Could you check a few things on this model? Use its own coordinates, in mm. A direction names the side the tool comes from. Give positions to 0.01 mm unless a question says otherwise; leave off trailing zeros. Loops run counter-clockwise (first coordinate to the right, second up) from the corner with the lowest first, then second, coordinate; pieces in that order, holes last. Notation, with made-up numbers: M 18,61.25 L 69,61.25 A9 cw 69,75.25 Z; hole C 2,-18 d7. An arc over 180 degrees is marked long. Write each question's results on one line, items separated by ' | '. Start each with the question number.
from build123d import *

# Parameters (mm, degrees)
SKETCH042_W     = 20
SKETCH042_H     = 20
PAD022_DEPTH    = 9
SKETCH043_R     = 7
PAD023_DEPTH    = 10
POCKET023_DEPTH = 8
SKETCH046_W     = 8.75
SKETCH046_H     = 5.2
POCKET024_DEPTH = 1
SKETCH047_R     = 3.7
POCKET025_DEPTH = 3
SKETCH048_R     = 1.675
POCKET026_DEPTH = 5
FILLET007_R     = 2
POCKET033_DEPTH = 5.2
SKETCH058_R     = 1.7
POCKET034_DEPTH = 10


with BuildPart() as part:
    # Sketch042 → Pad022 (new body)
    with BuildSketch(Plane.XZ):
        with Locations((-19.773271, -18.660706)):
            Rectangle(SKETCH042_W, SKETCH042_H)
    extrude(amount=PAD022_DEPTH)

    # Sketch043 (on Face6 of Pad022) → Pad023 (join)
    with BuildSketch(Plane.XZ.offset(9)):
        with Locations((-19.773271, -18.660706)):
            Circle(SKETCH043_R)
    extrude(amount=PAD023_DEPTH)

    # Sketch044 (on Face8 of Pad023) → Pocket023 (cut)
    with BuildSketch(Plane.XZ.offset(19)):
        with BuildLine():
            Line((-17.123271, -18.660706), (-17.123271, -31.745383))
            Line((-17.123271, -31.745383), (-22.423271, -31.745383))
            Line((-22.423271, -31.745383), (-22.423271, -18.660706))
            ThreePointArc((-17.123271, -18.660706), (-19.773271, -16.010706), (-22.423271, -18.660706))
        make_face()
    extrude(amount=-POCKET023_DEPTH, mode=Mode.SUBTRACT)

    # Sketch046 (on Face6 of Pocket023) → Pocket024 (cut)
    with BuildSketch(Plane(origin=(0, 0, -28.660706), x_dir=(1, 0, 0), z_dir=(0, 0, -1))):
        with Locations((-19.773271, 11.6)):
            Rectangle(SKETCH046_W, SKETCH046_H)
    extrude(amount=-POCKET024_DEPTH, mode=Mode.SUBTRACT)

    # Sketch047 (on Face4 of Pocket024) → Pocket025 (cut)
    with BuildSketch(Plane(origin=(0, 0, 0), x_dir=(1, 0, 0), z_dir=(0, 1, 0))):
        with Locations((-19.773271, 18.660706)):
            Circle(SKETCH047_R)
    extrude(amount=-POCKET025_DEPTH, mode=Mode.SUBTRACT)

    # Sketch048 (on Face11 of Pocket025) → Pocket026 (cut)
    with BuildSketch(Plane.XZ.offset(19)):
        with Locations((-19.773271, -18.660706)):
            Circle(SKETCH048_R)
    extrude(amount=-POCKET026_DEPTH, mode=Mode.SUBTRACT)

    # Fillet007
    fillet007_edges = [part.edges().sort_by_distance(p)[0] for p in [
        (-19.773271, 0, -8.660706),
        (-9.773271, 0, -18.660706),
        (-29.773271, 0, -18.660706),
        (-19.773271, 0, -28.660706),
        (-23.473271, 0, -18.660706),
        (-9.773271, -4.5, -28.660706),
        (-9.773271, -4.5, -8.660706),
        (-9.773271, -9, -18.660706),
        (-29.773271, -4.5, -28.660706),
        (-26.960771, -9, -28.660706),
        (-19.773271, -9, -28.660706),
        (-12.585771, -9, -28.660706),
        (-29.773271, -4.5, -8.660706),
        (-29.773271, -9, -18.660706),
        (-19.773271, -9, -8.660706),
    ]]
    fillet(fillet007_edges, radius=FILLET007_R)

    # Sketch057 (on Face32 of Fillet007) → Pocket033 (cut)
    with BuildSketch(Plane.XZ.offset(14.2)):
        with BuildLine():
            ThreePointArc((-15.373271, -18.660706), (-19.773271, -14.260706), (-24.173271, -18.660706))
            Line((-24.173271, -18.660706), (-24.173271, -31.35503))
            Line((-24.173271, -31.35503), (-15.373271, -31.35503))
            Line((-15.373271, -18.660706), (-15.373271, -31.35503))
        make_face()
    extrude(amount=-POCKET033_DEPTH, mode=Mode.SUBTRACT)

    # Sketch058 (on Face41 of Pocket033) → Pocket034 (cut)
    with BuildSketch(Plane(origin=(0, -3, 0), x_dir=(1, 0, 0), z_dir=(0, 1, 0))):
        with Locations((-19.773271, 18.660706)):
            Circle(SKETCH058_R)
    extrude(amount=-POCKET034_DEPTH, mode=Mode.SUBTRACT)


solid = part.part
1) If we section it at B-B on y = -8: Write out the boundary of the cut face in (x, z), plus the area to 3 significant figures.
2) I'm going to push flat-ended pins straight in: P1, Ø4, axis at y = -15, z = -17.5, coming from the -X side; P2, Ø8, axis at y = -16, z = -25, coming from the -X side; P3, Ø4, axis at y = -10.5, z = -20, coming from the -X side. Where does each tip first touch, or does it pass through?
3) Which directions (+Z, -Z, +X, -X, +Y, -Y) give clear straight access to the entire face, cutting with the end or side of a thin tool? Please do faces 1 (the face through (-20.58, -2.49, -15.05)), 2 (the face through (-17.123, -17, -22)), 3 (the face through (-19.68, -11.64, -14.26)).
4) If we section it at A-A on z = -9.75: Write out the boundary of the cut face in (x, y), plus the area to 3 significant figures.
5) Thinking about a two-plate mould opening in X: for faces 4 (the face through (-29.2, -4.54, -28.06)), 5 (the face through (-20, -19, -15)), 6 (the face through (-24.173, -12, -21)), which applies, pulls with the +X half, pulls with the -X half, needs draft (parallel to the pull), parting line crosses it, or undercut?
6) If we section it at C-C on x = -11.5: Write out the boundary of the cut face in (y, z).
7) If we section it at D-D on y = -11.5: Write out the boundary of the cut face in (x, z).
8) Please list where these lines run through material, in increasing order: line 1 (Y direction, x = -24, z = -23); line 2 (Y direction, x = -27.25, z = -19.25); line 3 (Y direction, x = -20.25, z = -20.5). Write a range as from..to.
Calculated:
1) outline: M -29.51,-26.66 A1.73 ccw -27.77,-28.39 L -11.77,-28.39 A1.73 ccw -10.04,-26.66 L -10.04,-10.66 A1.73 ccw -11.77,-8.93 L -27.77,-8.93 A1.73 ccw -29.51,-10.66 Z; hole C -19.77,-18.66 d3.4 | area: 367 mm2
2) P1: stops at x = -26.77 | P2: stops at x = -26.37 | P3: stops at x = -29.1
3) face 1: +Y | face 2: -Z, -Y | face 3: -Z
4) outline: M -29.55,-7 A1.78 ccw -27.77,-8.78 L -11.77,-8.78 A1.78 ccw -9.99,-7 L -9.99,-2 A1.78 ccw -11.77,-0.22 L -27.77,-0.22 A1.78 ccw -29.55,-2 Z | area: 165 mm2
5) face 4: pulls with the -X half | face 5: needs draft | face 6: undercut
6) outline: M -8.98,-26.66 A1.98 ccw -7,-28.64 L -2,-28.64 A1.98 ccw -0.02,-26.66 L -0.02,-10.66 A1.98 ccw -2,-8.68 L -7,-8.68 A1.98 ccw -8.98,-10.66 Z
7) outline: M -24.17,-24.1 L -24.17,-18.66 A4.4 cw -15.37,-18.66 L -15.37,-24.1 A7 ccw long Z
8) line 1: y = -19..-14.2, -9..0 | line 2: y = -9..0 | line 3: y = -9..-3
